```python
from build123d import *

# Parameters (mm, degrees)
BOSS_EXTRU_1_DEPTH = 3.3
ESQUISSE4_W        = 11.5
ESQUISSE4_H        = 3.35
BOSS_EXTRU_2_DEPTH = 1
ESQUISSE5_W        = 9.5
ESQUISSE5_H        = 3.35
BOSS_EXTRU_3_DEPTH = 0.7


with BuildPart() as part:
    # Esquisse3 → Boss.-Extru.1 (new body)
    with BuildSketch(Plane.XY):
        with BuildLine():
            Line((-2.7, 2.225), (2.7, 2.225))
            ThreePointArc((2.7, 2.225), (4.925, 0), (2.7, -2.225))
            Line((2.7, -2.225), (-2.7, -2.225))
            ThreePointArc((-2.7, -2.225), (-4.925, 0), (-2.7, 2.225))
        make_face()
    extrude(amount=BOSS_EXTRU_1_DEPTH)

    # Esquisse4 → Boss.-Extru.2 (add)
    with BuildSketch(Plane.XY.offset(3.3)):
        Rectangle(ESQUISSE4_W, ESQUISSE4_H)
    extrude(amount=BOSS_EXTRU_2_DEPTH)

    # Esquisse5 → Boss.-Extru.3 (add)
    with BuildSketch(Plane.XY.offset(4.3)):
        Rectangle(ESQUISSE5_W, ESQUISSE5_H)
    extrude(amount=BOSS_EXTRU_3_DEPTH)


solid = part.part
```
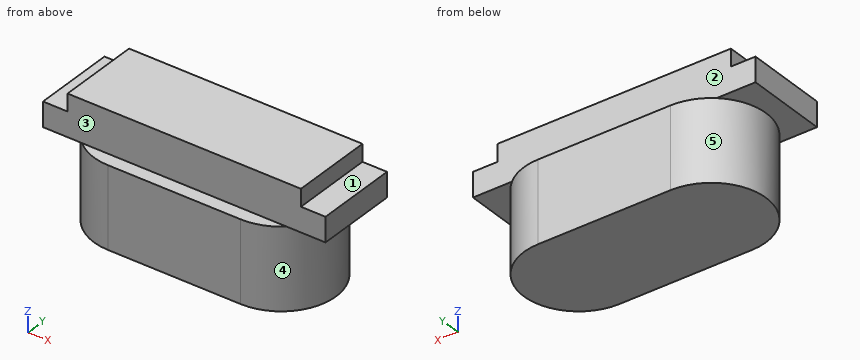
Work out the finished part from the listing and answer in its coordinate system (mm). Face numbers are marked on the shaded views. A direction names the side the tool comes from. Give positions to 0.01 mm unless a question says otherwise; leave off trailing zeros. Loops run counter-clockwise (first coordinate to the right, second up) from the corner with the lowest first, then second, coordinate; pieces in that order, holes last. Notation, with made-up numbers: (3.5, -13) - (23.5, -13) arc R22 ccw to (23.5, -3) - close; hole circle Ø9 at (-17.75, 87.5). An arc over 180 degrees is marked (long way). One line per question, with ' | ' between items.
(1) The part is cut by section A-A (y = 0). Write down the section's boundary in (x, z) (3 decimals), then the cut area to 3 significant figures.
Recorded:
outline: (-5.75, 3.3) - (-4.925, 3.3) - (-4.925, 0) - (4.925, 0) - (4.925, 3.3) - (5.75, 3.3) - (5.75, 4.3) - (4.75, 4.3) - (4.75, 5) - (-4.75, 5) - (-4.75, 4.3) - (-5.75, 4.3) - close | area: 50.7 mm²
(2) A tool of negligible diameter and unlimited length cuts with its end or side. For the marked faces 1, 2, 3, 4 and 5, from which of +Z, -Z, +X, -X, +Y, -Y can it reach the whole face along a straight path? Write none if from no direction.
Recorded:
face 1: +Z, +X, +Y, -Y | face 2: +Z, +X, -X, +Y | face 3: +Z, +X, -X, -Y | face 4: -Z, +X | face 5: -Z, -X
(3) Each of these flat-tipped pins is pushed along its axis until it touches: pin 1 Ø1.9 at (x, z) = (0.5, 4.5) entering from -Y (3 decimals); pin 2 Ø0.6 at (y, z) = (-0.5, 4.5) entering from -X; pin 3 Ø0.5 at (x, y) = (-5.5, -1) entering from +Z; pin 4 Ø0.8 at (x, z) = (1.5, 4) entering from +Y (3 decimals). Where does it stop, or does it pass through?
Recorded:
pin 1: stops at y = -1.675 | pin 2: stops at x = -5.75 | pin 3: stops at z = 4.3 | pin 4: stops at y = 1.675
(4) Straight lines are drawn through the part: probe 1 along Z at (x, y) = (5.25, 0); probe 2 along X at (y, z) = (-0.2, 4.8); probe 3 along Y at (x, z) = (1.75, 3.6) (3 decimals). For each, find the intervals that lie inside material, in ascending order.
Recorded:
probe 1: z = 3.3 to 4.3 | probe 2: x = -4.75 to 4.75 | probe 3: y = -1.675 to 1.675
(5) The part is cut by section B-B (x = 1.75). Write down the section's boundary in (y, z) (3 decimals).
Recorded:
outline: (-2.225, 0) - (2.225, 0) - (2.225, 3.3) - (1.675, 3.3) - (1.675, 5) - (-1.675, 5) - (-1.675, 3.3) - (-2.225, 3.3) - close
(6) The part is cut by section D-D (y = 1.15). Write down the section's boundary in (x, z), then the cut area to 3 significant figures.
Recorded:
outline: (-5.75, 3.3) - (-4.6, 3.3) - (-4.6, 0) - (4.6, 0) - (4.6, 3.3) - (5.75, 3.3) - (5.75, 4.3) - (4.75, 4.3) - (4.75, 5) - (-4.75, 5) - (-4.75, 4.3) - (-5.75, 4.3) - close | area: 48.5 mm²
(7) The part is cut by section C-C (z = 4.1). Write down the section's boundary in (x, y) (3 decimals).
Recorded:
outline: (-5.75, -1.675) - (5.75, -1.675) - (5.75, 1.675) - (-5.75, 1.675) - close
